Could you check a few things on this model? Use its own coordinates, in mm. Face numbers are marked on the shaded views. Round coordinates to 2 decimals unless told otherwise and drop trailing zeros. Loops run counter-clockwise (first coordinate to the right, second up) from the corner with the lowest first, then second, coordinate; pieces in that order, holes last. Notation, with made-up numbers: (-6, 29) -> (-2, 29) arc R24 ccw to (-2, 45) -> close; hole circle Ø6 at (28, 13.25). An arc over 180 degrees is marked (long way). One line per item, written item: value.
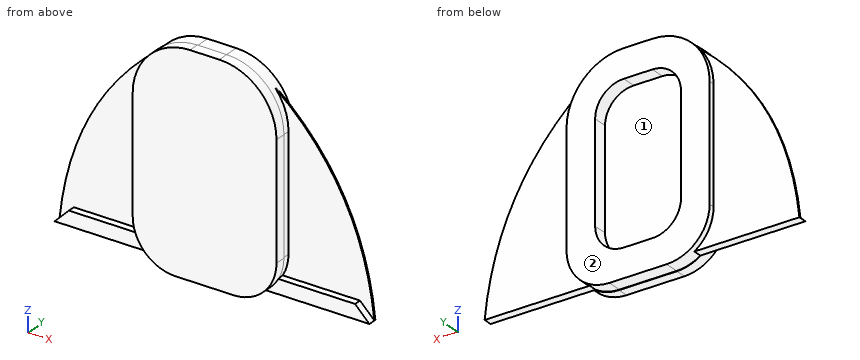
```python
from build123d import *

# Parameters (mm, degrees)
EXTRUDE_1_DEPTH = 1.5
SKETCH_2_W      = 2
SKETCH_2_H      = 22
EXTRUDE_2_DEPTH = 1
EXTRUDE_3_DEPTH = 0.2
EXTRUDE_4_DEPTH = 2


with BuildPart() as part:
    # 草图1 → 凸台-拉伸1 (new body)
    with BuildSketch(Plane(origin=(0, 0, 0), x_dir=(1, 0, 0), z_dir=(0, 1, 0))):
        with BuildLine():
            Line((-4.05, 15.05), (4.05, 15.05))
            ThreePointArc((4.05, 15.05), (8.292640687, 13.292640687), (10.05, 9.05))
            Line((10.05, 9.05), (10.05, -7.05))
            ThreePointArc((10.05, -7.05), (7.706854249, -12.706854249), (2.05, -15.05))
            Line((2.05, -15.05), (-2.05, -15.05))
            ThreePointArc((-2.05, -15.05), (-7.706854249, -12.706854249), (-10.05, -7.05))
            Line((-10.05, -7.05), (-10.05, 9.05))
            ThreePointArc((-10.05, 9.05), (-8.292640687, 13.292640687), (-4.05, 15.05))
        make_face()
    extrude(amount=EXTRUDE_1_DEPTH)

    # 草图2 → 凸台-拉伸2 (add)
    with BuildSketch(Plane(origin=(0, 1.5, 0), x_dir=(1, 0, 0), z_dir=(0, 1, 0))):
        with Locations((-8, 1)):
            Rectangle(SKETCH_2_W, SKETCH_2_H)
        with BuildLine():
            Line((-9, 12), (-7, 12))
            Line((-7, 12), (-2, 12))
            Line((-2, 12), (-2, 14))
            Line((-2, 14), (-7.440796367, 14))
            ThreePointArc((-7.440796367, 14), (-8.472295614, 13.105034094), (-9.274700948, 12))
            Line((-9.274700948, 12), (-9, 12))
        make_face()
        with BuildLine():
            Line((-20, 12), (-9.274700948, 12))
            ThreePointArc((-9.274700948, 12), (-8.472295614, 13.105034094), (-7.440796367, 14))
            Line((-7.440796367, 14), (-20, 14))
            Line((-20, 14), (-20, 12))
        make_face()
        Polygon((-20, 14), (-22, 14), (-20, 12), align=None)
        Polygon((-7, -13), (-9, -10), (-7, -10), align=None)
        with BuildLine():
            ThreePointArc((9.274700948, 12), (8.472295614, 13.105034094), (7.440796367, 14))
            Line((7.440796367, 14), (2, 14))
            Line((2, 14), (2, 12))
            Line((2, 12), (7, 12))
            Line((7, 12), (9, 12))
            Line((9, 12), (9.274700948, 12))
        make_face()
        with BuildLine():
            Line((20, 12), (20, 14))
            Line((20, 14), (7.440796367, 14))
            ThreePointArc((7.440796367, 14), (8.472295614, 13.105034094), (9.274700948, 12))
            Line((9.274700948, 12), (20, 12))
        make_face()
        Polygon((20, 12), (20, 14), (22, 14), align=None)
        with Locations((8, 1)):
            Rectangle(SKETCH_2_W, SKETCH_2_H)
        Polygon((7, -10), (9, -10), (7, -13), align=None)
    extrude(amount=EXTRUDE_2_DEPTH)

    # 草图3 → 凸台-拉伸3 (add)
    with BuildSketch(Plane(origin=(0, 2.5, 0), x_dir=(1, 0, 0), z_dir=(0, 1, 0))):
        with BuildLine():
            Line((-7, -13), (-7, 14))
            Line((-7, 14), (-22, 14))
            add(Edge.make_bspline(
                [(-22, 14), (-20.203305703, -3.149159716), (-7, -13)],
                knots=[0, 0, 0, 1, 1, 1], degree=2))
        make_face()
        with BuildLine():
            Line((7, -13), (7, 14))
            Line((7, 14), (22, 14))
            add(Edge.make_bspline(
                [(22, 14), (20.203305703, -3.149159716), (7, -13)],
                knots=[0, 0, 0, 1, 1, 1], degree=2))
        make_face()
    extrude(amount=EXTRUDE_3_DEPTH)

    # 草图4 → 凸台-拉伸4 (add)
    with BuildSketch(Plane(origin=(0, 1.5, 0), x_dir=(1, 0, 0), z_dir=(0, 1, 0))):
        with BuildLine():
            Line((-4, 15), (4, 15))
            ThreePointArc((4, 15), (8.242640687, 13.242640687), (10, 9))
            Line((10, 9), (10, -7))
            ThreePointArc((10, -7), (7.656854249, -12.656854249), (2, -15))
            Line((2, -15), (-2, -15))
            ThreePointArc((-2, -15), (-7.656854249, -12.656854249), (-10, -7))
            Line((-10, -7), (-10, 9))
            ThreePointArc((-10, 9), (-8.242640687, 13.242640687), (-4, 15))
        make_face()
        with BuildLine():
            Line((-2, 11), (2, 11))
            ThreePointArc((2, 11), (4.828427125, 9.828427125), (6, 7))
            Line((6, 7), (6, -7))
            ThreePointArc((6, -7), (4.828427125, -9.828427125), (2, -11))
            Line((2, -11), (-2, -11))
            ThreePointArc((-2, -11), (-4.828427125, -9.828427125), (-6, -7))
            Line((-6, -7), (-6, 7))
            ThreePointArc((-6, 7), (-4.828427125, 9.828427125), (-2, 11))
        make_face(mode=Mode.SUBTRACT)
    extrude(amount=EXTRUDE_4_DEPTH)


solid = part.part
```
Item 1: I need wall thicknesses on line 1 (X direction, y = 2.1, z = -3); line 2 (Z direction, x = 5, y = 3.1); line 3 (X direction, y = 2.9, z = 9). Which ranges of each line are inside material? Lowest first, please. Write a range as from..to.
Output:
line 1: x = -10..-6, 6..10
line 2: z = -14.92..-9.65, 9.65..14.42
line 3: x = -9.75..-5.46, 5.46..9.75
Item 2: If we mould it in two halves opening along X, with no side actions, what happens to the marked faces 1 and 2? For each: released by +X, released by -X, zero draft, split by the parting line, or undercut.
Output:
face 1: undercut
face 2: zero draft
Item 3: Will these pins go through, and if not, where does the flat tip stop? pin 1 Ø4.5 at (x, z) = (16.5, 0.5) entering from +Y; pin 2 Ø1.5 at (x, y) = (5, 2.5) entering from +Z; pin 3 Ø2 at (x, z) = (-12.5, -13.5) entering from -Y.
Output:
pin 1: stops at y = 2.7
pin 2: stops at z = 14.68
pin 3: stops at y = 1.5
Item 4: If we section it at A-A on x = 1.5: List the corners of the cut face in (y, z) for me, plus the area to 4 significant figures.
Output:
outline: (0, -15.05) -> (1.5, -15.05) -> (1.5, -15) -> (3.5, -15) -> (3.5, -11) -> (1.5, -11) -> (1.5, 11) -> (3.5, 11) -> (3.5, 15) -> (1.5, 15) -> (1.5, 15.05) -> (0, 15.05) -> close
area: 61.15 mm²
